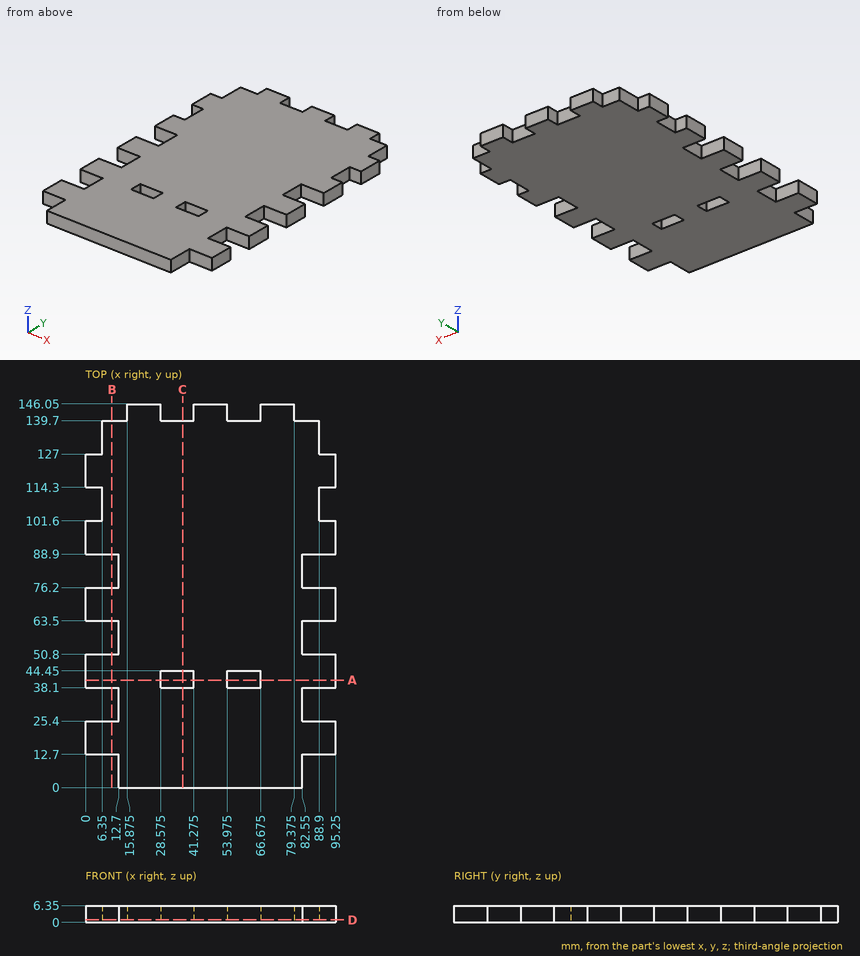
Job drawing, mm, ordinate dimensions from the low corner. One solid piece. Round coordinates to 2 decimals unless told otherwise and drop trailing zeros. Write each loop counter-clockwise with the first axis right and the second up, starting at its lowest first coordinate (ties: lowest second). Pieces come first, ordered by that corner, then holes.
1) Band-saw the part on D-D, the plane z = 1. Give the number of separate pieces and of enclosed holes in the cut face, and give its area (3 significant figures).
2) Band-saw the part on B-B, the plane x = 10. List the corners of the cut face in (y, z).
3) Drill centre lines: probe 1 along Y at (x, z) = (10.5, 3); probe 2 along Y at (x, z) = (90, 1); probe 3 along Y at (x, z) = (37, 2.75). Where is each one in solid material? Low to high.
4) Pin check, flat tips, straight feed: pin 1 (10 mm diameter, centred on x = 46, y = 66.5, fed in from -Z); pin 2 (3 mm diameter, centred on y = 143, z = 3.5, fed in from -X) (3 decimals); pin 3 (3 mm diameter, centred on x = 5, z = 4, fed in from -Y); pin 4 (1 mm diameter, centred on x = 64.5, z = 3, fed in from +Y). Stop position of each tip, or through.
5) Band-saw the part on A-A, the plane y = 41. List the corners of the cut face in (x, z) (3 decimals), and give its area (3 significant figures).
6) Band-saw the part on C-C, the plane x = 37. List the corners of the cut face in (y, z), and give its area (3 significant figures).
Ans:
1. separate pieces: 1
1. enclosed holes: 2
1. area: 11,800 mm2
2. outline: (12.7, 0) - (25.4, 0) - (25.4, 6.35) - (12.7, 6.35) - close; (38.1, 0) - (50.8, 0) - (50.8, 6.35) - (38.1, 6.35) - close; (63.5, 0) - (76.2, 0) - (76.2, 6.35) - (63.5, 6.35) - close; (88.9, 0) - (139.7, 0) - (139.7, 6.35) - (88.9, 6.35) - close
3. probe 1: y = 12.7 to 25.4, 38.1 to 50.8, 63.5 to 76.2, 88.9 to 139.7
3. probe 2: y = 12.7 to 25.4, 38.1 to 50.8, 63.5 to 76.2, 88.9 to 101.6, 114.3 to 127
3. probe 3: y = 0 to 38.1, 44.45 to 139.7
4. pin 1: stops at z = 0
4. pin 2: stops at x = 15.875
4. pin 3: stops at y = 12.7
4. pin 4: stops at y = 139.7
5. outline: (0, 0) - (28.575, 0) - (28.575, 6.35) - (0, 6.35) - close; (41.275, 0) - (53.975, 0) - (53.975, 6.35) - (41.275, 6.35) - close; (66.675, 0) - (95.25, 0) - (95.25, 6.35) - (66.675, 6.35) - close
5. area: 444 mm2
6. outline: (0, 0) - (38.1, 0) - (38.1, 6.35) - (0, 6.35) - close; (44.45, 0) - (139.7, 0) - (139.7, 6.35) - (44.45, 6.35) - close
6. area: 847 mm2
